Build history of the part. All positions in model axes, mm. Face numbers are marked on the shaded views. Coordinates: 2 decimals unless noted, no trailing zeros. Loops run counter-clockwise (first coordinate to the right, second up) from the corner with the lowest first, then second, coordinate; pieces in that order, holes last.
Item 1: Flat gauge pins, fed straight in: pin 1 (10 mm diameter, centred on y = 6, z = 52.5, fed in from -X); pin 2 (5.5 mm diameter, centred on x = 2.5, y = -2, fed in from -Z); pin 3 (10 mm diameter, centred on x = -25, y = 5.5, fed in from -Z) (3 decimals). Where does each tip first touch, or does it go through?
Item 2: Cut at D-D (z = 118.5). List the corners of the cut face in (x, y), and give its area (3 significant figures).
Item 3: Drill centre lines: line 1 along Y through (x, z) = (0, 76); line 2 along Z through (x, y) = (-46.5, -13) (3 decimals); line 3 along X through (y, z) = (-3.5, 35.5). Where is each one in solid material? Low to high.
Item 4: Cut at A-A (x = 0). List the corners of the cut face in (y, z) (3 decimals).
Item 5: Cut at C-C (z = 163.5). List the corners of the cut face in (x, y).
Item 6: Cut at B-B (y = 0). List the corners of the cut face in (x, z) (3 decimals).
Item 7: Mould opens along Z. For the marked faces 1, 2, 3 and 4 say: released by +Z, released by -Z, zero draft, split by the parting line, or undercut.
from build123d import *

# Parameters (mm, degrees)
SKETCH2_R           = 15.875
BOSS_EXTRUDE1_DEPTH = 44.45
SKETCH3_R           = 12.7
BOSS_EXTRUDE2_DEPTH = 113.665
SKETCH4_R           = 11.01725
BOSS_EXTRUDE3_DEPTH = 38.1
SKETCH6_R           = 5.55625
CUT_EXTRUDE1_DEPTH  = 215.9
SKETCH8_W           = 157.285598566
SKETCH8_H           = 178.663022366
BOSS_EXTRUDE5_DEPTH = 9.525


with BuildPart() as part:
    # Sketch2 → Boss-Extrude1 (new body)
    with BuildSketch(Plane.XY):
        Circle(SKETCH2_R)
    extrude(amount=BOSS_EXTRUDE1_DEPTH)

    # Sketch3 → Boss-Extrude2 (add)
    with BuildSketch(Plane.XY.offset(44.45)):
        Circle(SKETCH3_R)
    extrude(amount=BOSS_EXTRUDE2_DEPTH)

    # Sketch4 → Boss-Extrude3 (add)
    with BuildSketch(Plane.XY.offset(158.115)):
        Circle(SKETCH4_R)
    extrude(amount=BOSS_EXTRUDE3_DEPTH)

    # Sketch6 → Cut-Extrude1 (cut)
    with BuildSketch(Plane(origin=(0, 0, 0), x_dir=(-1, 0, 0), z_dir=(0, 0, -1))):
        Circle(SKETCH6_R)
    extrude(amount=-CUT_EXTRUDE1_DEPTH, mode=Mode.SUBTRACT)

    # Sketch8 → Boss-Extrude5 (add)
    with BuildSketch(Plane.XY.offset(196.215)):
        Rectangle(SKETCH8_W, SKETCH8_H)
    extrude(amount=BOSS_EXTRUDE5_DEPTH)


solid = part.part
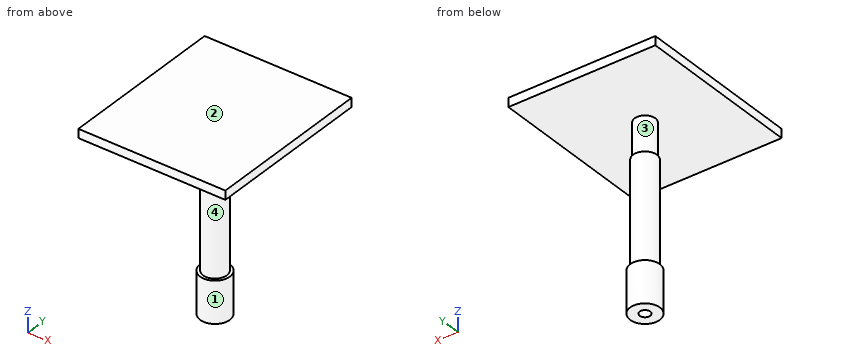
Filled sheet:
1. pin 1: stops at x = -12.66
1. pin 2: stops at z = 0
1. pin 3: stops at z = 196.215
2. outline: circle Ø25.4 at (0, 0); hole circle Ø11.11 at (0, 0)
2. area: 410 mm2
3. line 1: y = -12.7 to -5.56, 5.56 to 12.7
3. line 2: z = 196.215 to 205.74
3. line 3: x = -15.48 to -4.32, 4.32 to 15.48
4. outline: (-89.332, 196.215) - (-11.017, 196.215) - (-11.017, 158.115) - (-12.7, 158.115) - (-12.7, 44.45) - (-15.875, 44.45) - (-15.875, 0) - (-5.556, 0) - (-5.556, 196.215) - (5.556, 196.215) - (5.556, 0) - (15.875, 0) - (15.875, 44.45) - (12.7, 44.45) - (12.7, 158.115) - (11.017, 158.115) - (11.017, 196.215) - (89.332, 196.215) - (89.332, 205.74) - (-89.332, 205.74) - close
5. outline: circle Ø22.03 at (0, 0); hole circle Ø11.11 at (0, 0)
6. outline: (-78.643, 196.215) - (-11.017, 196.215) - (-11.017, 158.115) - (-12.7, 158.115) - (-12.7, 44.45) - (-15.875, 44.45) - (-15.875, 0) - (-5.556, 0) - (-5.556, 196.215) - (5.556, 196.215) - (5.556, 0) - (15.875, 0) - (15.875, 44.45) - (12.7, 44.45) - (12.7, 158.115) - (11.017, 158.115) - (11.017, 196.215) - (78.643, 196.215) - (78.643, 205.74) - (-78.643, 205.74) - close
7. face 1: zero draft
7. face 2: released by +Z
7. face 3: undercut
7. face 4: undercut
